Could you check a few things on this model? Use its own coordinates, in mm. Give positions to 0.01 mm unless a question says otherwise; leave off trailing zeros. Loops run counter-clockwise (first coordinate to the right, second up) from the corner with the lowest first, then second, coordinate; pieces in that order, holes last. Notation, with made-up numbers: (49, 2) - (66, 2) arc R18 ccw to (66, 31) - close; hole circle Ø2 at (88.25, -22.5). An arc over 180 degrees is marked (long way). One line per item, written item: value. Start each with the question number.
Q1. I want a section at B-B (x = 65.85). Please give me the cut outline in (y, z).
Q2. If I drill on line 1 (Y direction, x = 65.7, z = 17); line 2 (Z direction, x = 65.4, y = 16); line 3 (Z direction, x = 65.6, y = 18.5), over which ranges is the centre line in solid material (lowest first)? Write a range as from..to.
Q3. I want a section at A-A (z = 32). Please give me the cut outline in (x, y), then the cut area to 3 significant figures.
Q4. I want a section at C-C (z = 17). Please give me the cut outline in (x, y), then the cut area to 3 significant figures.
```python
from build123d import *

# Parameters (mm, degrees)
EKSTR_ZYON_NCE1_DEPTH = 50
IZIM2_R               = 3
KES_EKSTR_ZYON1_DEPTH = 78
IZIM3_R               = 0.5
KES_EKSTR_ZYON2_DEPTH = 22
IZIM4_R               = 6
KES_EKSTR_ZYON3_DEPTH = 22
SCALE1_SCALE          = 0.666666667
SKETCH3_W             = 33.333333334
SKETCH3_H             = 19.333333333
CUT_EXTRUDE1_DEPTH    = 2
SKETCH4_W             = 56
SKETCH4_H             = 55
BOSS_EXTRUDE1_DEPTH   = 2
SKETCH5_W             = 33.333333334
SKETCH5_H             = 18
BOSS_EXTRUDE2_DEPTH   = 1.5
SKETCH6_R             = 2
CUT_EXTRUDE2_DEPTH    = 1.5
SKETCH7_W             = 56.964320229
SKETCH7_H             = 23.03419096
CUT_EXTRUDE5_DEPTH    = 56
SKETCH8_W             = 56.142360806
SKETCH8_H             = 4.377004861
CUT_EXTRUDE6_DEPTH    = 2.5


with BuildPart() as part:
    # Çizim1 → Ekstrüzyon-İnce1 (new body)
    with BuildSketch(Plane.XY):
        with BuildLine():
            Line((0, 0), (0, 29))
            ThreePointArc((0, 29), (0.292893219, 29.707106781), (1, 30))
            Line((1, 30), (57, 30))
            ThreePointArc((57, 30), (57.707106781, 29.707106781), (58, 29))
            Line((58, 29), (58, 0))
            Line((58, 0), (57, 0))
            Line((57, 0), (57, 29))
            Line((57, 29), (1, 29))
            Line((1, 29), (1, 0))
            Line((1, 0), (0, 0))
        make_face()
    extrude(amount=EKSTR_ZYON_NCE1_DEPTH)

    # Çizim2 → Kes-Ekstrüzyon1 (cut)
    with BuildSketch(Plane(origin=(58, 0, 0), x_dir=(0, 0, -1), z_dir=(1, 0, 0))):
        with Locations((-36.75, 14.5)):
            Circle(IZIM2_R)
        with Locations((-13.25, 14.5)):
            Circle(IZIM2_R)
    extrude(amount=-KES_EKSTR_ZYON1_DEPTH, mode=Mode.SUBTRACT)

    # Çizim3 → Kes-Ekstrüzyon2 (cut)
    with BuildSketch(Plane.ZY):
        with Locations((46.926319902, 2.636193895)):
            Circle(IZIM3_R)
    extrude(amount=-KES_EKSTR_ZYON2_DEPTH, mode=Mode.SUBTRACT)

    # Çizim4 → Kes-Ekstrüzyon3 (cut)
    with BuildSketch(Plane.ZY):
        with Locations((36.75, 14.5)):
            Circle(IZIM4_R)
    extrude(amount=-KES_EKSTR_ZYON3_DEPTH, mode=Mode.SUBTRACT)


with BuildPart() as part_1:
    # Scale1: scaled about (29.437260205, 22.238846327, 24.818293672)
    add(part.part.scale(SCALE1_SCALE).moved(Location((9.812420068, 7.412948776, 8.272764557))))

    # Sketch3 → Cut-Extrude1 (cut)
    with BuildSketch(Plane(origin=(48.479086735, 0, 0), x_dir=(0, 0, -1), z_dir=(1, 0, 0))):
        with Locations((-24.939431224, 17.079615442)):
            Rectangle(SKETCH3_W, SKETCH3_H)
    extrude(amount=-CUT_EXTRUDE1_DEPTH, mode=Mode.SUBTRACT)

    # Sketch4 → Boss-Extrude1 (add)
    with BuildSketch(Plane(origin=(0, 27.412948776, 0), x_dir=(1, 0, 0), z_dir=(0, 1, 0))):
        with Locations((38.479086736, -24.938368242)):
            Rectangle(SKETCH4_W, SKETCH4_H)
    extrude(amount=-BOSS_EXTRUDE1_DEPTH)

    # Sketch5 → Boss-Extrude2 (add)
    with BuildSketch(Plane(origin=(66.479086736, 0, 0), x_dir=(0, 0, -1), z_dir=(1, 0, 0))):
        with Locations((-24.939431224, 16.412948776)):
            Rectangle(SKETCH5_W, SKETCH5_H)
    extrude(amount=-BOSS_EXTRUDE2_DEPTH)

    # Sketch6 → Cut-Extrude2 (cut)
    with BuildSketch(Plane.ZY.offset(-64.979086736)):
        with Locations((17.106097891, 17.079615442)):
            Circle(SKETCH6_R)
        with Locations((32.772764557, 17.079615442)):
            Circle(SKETCH6_R)
    extrude(amount=-CUT_EXTRUDE2_DEPTH, mode=Mode.SUBTRACT)

    # Sketch7 → Cut-Extrude5 (cut, through all)
    with BuildSketch(Plane(origin=(0, 0, -2.561631758), x_dir=(-1, 0, 0), z_dir=(0, 0, -1))):
        with Locations((-36.496926622, 18.930044256)):
            Rectangle(SKETCH7_W, SKETCH7_H)
    extrude(amount=-CUT_EXTRUDE5_DEPTH, mode=Mode.SUBTRACT)

    # Sketch8 → Cut-Extrude6 (cut, through all)
    with BuildSketch(Plane.ZY.offset(-64.979086736)):
        with Locations((24.367187839, 27.601451207)):
            Rectangle(SKETCH8_W, SKETCH8_H)
    extrude(amount=-CUT_EXTRUDE6_DEPTH, mode=Mode.SUBTRACT)


solid = part_1.part
```
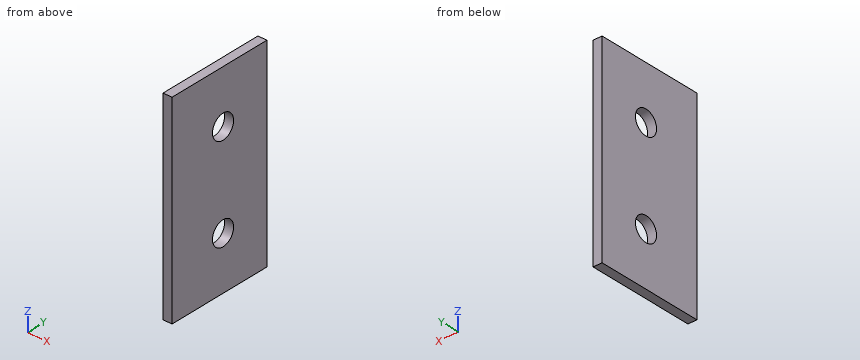
Worked answers:
1. outline: (7.41, 8.27) - (25.41, 8.27) - (25.41, 41.61) - (7.41, 41.61) - close; hole circle Ø4 at (17.08, 17.11); hole circle Ø4 at (17.08, 32.77)
2. line 1: y = 7.41..15.08, 19.08..25.41
2. line 2: z = 8.27..15.42, 18.79..31.09, 34.46..41.61
2. line 3: z = 8.27..15.7, 18.51..31.36, 34.18..41.61
3. outline: (64.98, 7.41) - (66.48, 7.41) - (66.48, 15.23) - (64.98, 15.23) - close; (64.98, 18.92) - (66.48, 18.92) - (66.48, 25.41) - (64.98, 25.41) - close
3. area: 21.5 mm²
4. outline: (64.98, 7.41) - (66.48, 7.41) - (66.48, 15.08) - (64.98, 15.08) - close; (64.98, 19.08) - (66.48, 19.08) - (66.48, 25.41) - (64.98, 25.41) - close
4. area: 21.0 mm²
